Autodesk Inventor part; units mm, degrees
ref_plane "YZ Plane" through (0, 0, 0) normal (1, 0, 0) x (0, 1, 0)
ref_plane "XZ Plane" through (0, 0, 0) normal (0, 1, 0) x (-1, 0, 0)
ref_plane "XY Plane" through (0, 0, 0) normal (0, 0, 1) x (1, 0, 0)
sketch "Skizze1" plane through (0, 0, 0) normal (0, 0, 1) x (1, 0, 0)
  circle A0 centre (0, 13) radius 1.25
  circle A1 centre (0, -13) radius 1.25
  circle A2 centre (11.2583, 6.5) radius 1.25
  circle A3 centre (11.2583, -6.5) radius 1.25
  circle A4 centre (-11.2583, 6.5) radius 1.25
  circle A5 centre (-11.2583, -6.5) radius 1.25
  arc A6 (-8.7265, -12.2003) -> (-6.2025, -13.6575) centre (0, 0) ccw
  arc A7 (-8.9067, -9.0923) -> (-8.7265, -12.2003) centre (-7.563, -10.5736) ccw
  arc A8 (-8.9067, -9.0923) -> (-12.3275, -3.1673) centre (-11.2583, -6.5) ccw
  arc A9 (-14.929, -1.4572) -> (-12.3275, -3.1673) centre (-12.9385, -1.2629) ccw
  arc A10 (-14.929, 1.4572) -> (-14.929, -1.4572) centre (0, 0) ccw
  arc A11 (-12.3275, 3.1673) -> (-14.929, 1.4572) centre (-12.9385, 1.2629) ccw
  arc A12 (-12.3275, 3.1673) -> (-8.9067, 9.0923) centre (-11.2583, 6.5) ccw
  arc A13 (-8.7265, 12.2003) -> (-8.9067, 9.0923) centre (-7.563, 10.5736) ccw
  arc A14 (-6.2025, 13.6575) -> (-8.7265, 12.2003) centre (0, 0) ccw
  arc A15 (-3.4208, 12.2596) -> (-6.2025, 13.6575) centre (-5.3755, 11.8365) ccw
  arc A16 (-3.4208, 12.2596) -> (3.4208, 12.2596) centre (0, 13) ccw
  arc A17 (6.2025, 13.6575) -> (3.4208, 12.2596) centre (5.3755, 11.8365) ccw
  arc A18 (8.7265, 12.2003) -> (6.2025, 13.6575) centre (0, 0) ccw
  arc A19 (8.9067, 9.0923) -> (8.7265, 12.2003) centre (7.563, 10.5736) ccw
  arc A20 (8.9067, 9.0923) -> (12.3275, 3.1673) centre (11.2583, 6.5) ccw
  arc A21 (14.929, 1.4572) -> (12.3275, 3.1673) centre (12.9385, 1.2629) ccw
  arc A22 (14.929, -1.4572) -> (14.929, 1.4572) centre (0, 0) ccw
  arc A23 (12.3275, -3.1673) -> (14.929, -1.4572) centre (12.9385, -1.2629) ccw
  arc A24 (12.3275, -3.1673) -> (8.9067, -9.0923) centre (11.2583, -6.5) ccw
  arc A25 (8.7265, -12.2003) -> (8.9067, -9.0923) centre (7.563, -10.5736) ccw
  arc A26 (6.2025, -13.6575) -> (8.7265, -12.2003) centre (0, 0) ccw
  arc A27 (3.4208, -12.2596) -> (6.2025, -13.6575) centre (5.3755, -11.8365) ccw
  arc A28 (3.4208, -12.2596) -> (-3.4208, -12.2596) centre (0, -13) ccw
  arc A29 (-6.2025, -13.6575) -> (-3.4208, -12.2596) centre (-5.3755, -11.8365) ccw
  circle A30 centre (0, 0) radius 17.5
  circle A31 centre (0, 0) radius 19.42
  circle A32 centre (0, 0) radius 3
  point P0 (0, 0)
  dimension "d0" = 6
extrude "Extrusion1" add sketch "Skizze1" along normal blind 3 contours A7 A8 A9 A10 A11 A12 A13 A14 A15 A16 A17 A18 A19 A20 A21 A22 A23 A24 A25 A26 A27 A28 A29 A6 | A30 | A31
sketch "Skizze2" plane through (0, 0, 3) normal (0, 0, 1) x (1, 0, 0)
  circle A0 centre (0, 0) radius 3
  circle A1 centre (-11.2583, -6.5) radius 1.25
  circle A2 centre (-11.2583, 6.5) radius 1.25
  circle A3 centre (11.2583, -6.5) radius 1.25
  circle A4 centre (11.2583, 6.5) radius 1.25
  circle A5 centre (0, -13) radius 1.25
  circle A6 centre (0, 13) radius 1.25
  circle A7 centre (0, 0) radius 19.42
  point P0 (0, 0)
hole "Bohrung1" at (-11.2583, 6.5, 3) at (0, -13, 3) at (11.2583, 6.5, 3) direction (0, 0, -1) diameter 3 end through all countersink diameter 6 countersink angle 90
properties part number "GripperMountCover" material "ABS-Kunststoff"
The model under review builds one solid part; all positions refer to its coordinate system, in mm. Give positions to 0.01 mm unless a question says otherwise; leave off trailing zeros. Write each loop counter-clockwise with the first axis right and the second up, starting at its lowest first coordinate (ties: lowest second). Pieces come first, ordered by that corner, then holes. Notation, with made-up numbers: (-10.5, 43) -> (-6.5, 43) arc R26 cw to (-6.5, 57) -> close; hole circle Ø7 at (75.25, -34.5). An arc over 180 degrees is marked (long way). Put each result on its own line as item: value.
(1) We need section D-D, the plane y = 13. Give the boundary of the cut face in (x, z), and give its area (3 significant figures).
Results are:
outline: (-14.43, 0) -> (-1.25, 0) -> (-1.25, 3) -> (-14.43, 3) -> close; (1.25, 0) -> (14.43, 0) -> (14.43, 3) -> (1.25, 3) -> close
area: 79.1 mm²
(2) We need section A-A, the plane y = 0. Give the boundary of the cut face in (x, z), and give its area (3 significant figures).
Results are:
outline: (-19.42, 0) -> (-3, 0) -> (-3, 3) -> (-19.42, 3) -> close; (3, 0) -> (19.42, 0) -> (19.42, 3) -> (3, 3) -> close
area: 98.5 mm²
(3) We need section C-C, the plane y = 6.5. Give the boundary of the cut face in (x, z).
Results are:
outline: (-18.3, 0) -> (-12.76, 0) -> (-12.76, 1.5) -> (-14.26, 3) -> (-18.3, 3) -> close; (-9.76, 0) -> (9.76, 0) -> (9.76, 1.5) -> (8.26, 3) -> (-8.26, 3) -> (-9.76, 1.5) -> close; (12.76, 0) -> (18.3, 0) -> (18.3, 3) -> (14.26, 3) -> (12.76, 1.5) -> close
(4) To check wall thickness, follow probe 1 along Y at (x, z) = (0, 1.1); probe 2 along X at (y, z) = (5, 1.95); probe 3 along X at (y, z) = (6.5, 0.5). State the ranges of each line that lie inside material, in increasing order. Write a range as from..to.
Results are:
probe 1: -19.42..-14.5, -11.5..-3, 3..11.75, 14.25..19.42
probe 2: -18.77..-12.5, -10.01..10.01, 12.5..18.77
probe 3: -18.3..-12.76, -9.76..9.76, 12.76..18.3
(5) For pin 1 Ø1.5 at (x, z) = (0, 0.5) entering from -Y; pin 2 Ø1.8 at (x, y) = (0, -13) entering from -Z; pin 3 Ø1.5 at (x, z) = (11.5, 1.5) entering from +Y; pin 4 Ø1.5 at (x, z) = (-10.5, 0.5) entering from -Y, all flat-tipped, find the tip position at first contact; note any pin that passes through.
Results are:
pin 1: y = -19.42
pin 2: through
pin 3: y = 16.17
pin 4: y = -16.8
(6) The part is to be moulded in two halves that separate along Y. For faces 1 (the flat face through (0, -4, 3)), 2 (the cylindrical face through (17.94, 7.44, 1.48)), 3 (the cylindrical face through (10.3, -5.7, 1.5)), say which applies: pulls with the +Y half, pulls with the -Y half, needs draft (parallel to the pull), parting line crosses it, or undercut.
Results are:
face 1: needs draft
face 2: parting line crosses it
face 3: undercut
(7) We need section B-B, the plane z = 0.65. Give the boundary of the cut face in (x, y).
Results are:
outline: circle Ø38.84 at (0, 0); hole circle Ø3 at (-11.26, 6.5); hole circle Ø2.5 at (-11.26, -6.5); hole circle Ø6 at (0, 0); hole circle Ø3 at (0, -13); hole circle Ø2.5 at (0, 13); hole circle Ø3 at (11.26, 6.5); hole circle Ø2.5 at (11.26, -6.5)
